The figure shows three views and two pictorial views of one solid part (mm, origin at its lowest corner). Answer the questions. A direction names the side the tool comes from. Coordinates: 2 decimals unless noted, no trailing zeros. Order: outer loops, then holes, each group sorted by start corner. A loop starts at its lowest first (then second) coordinate and runs counter-clockwise, first axis right, second up. Notation, with made-up numbers: (38, 80.5) - (54, 80.5) arc R18 cw to (54, 100.5) - close; hole circle Ø5 at (17.25, 86.25). An arc over 180 degrees is marked (long way). Answer as a JSON object with one key per item and string values. Group by question number.
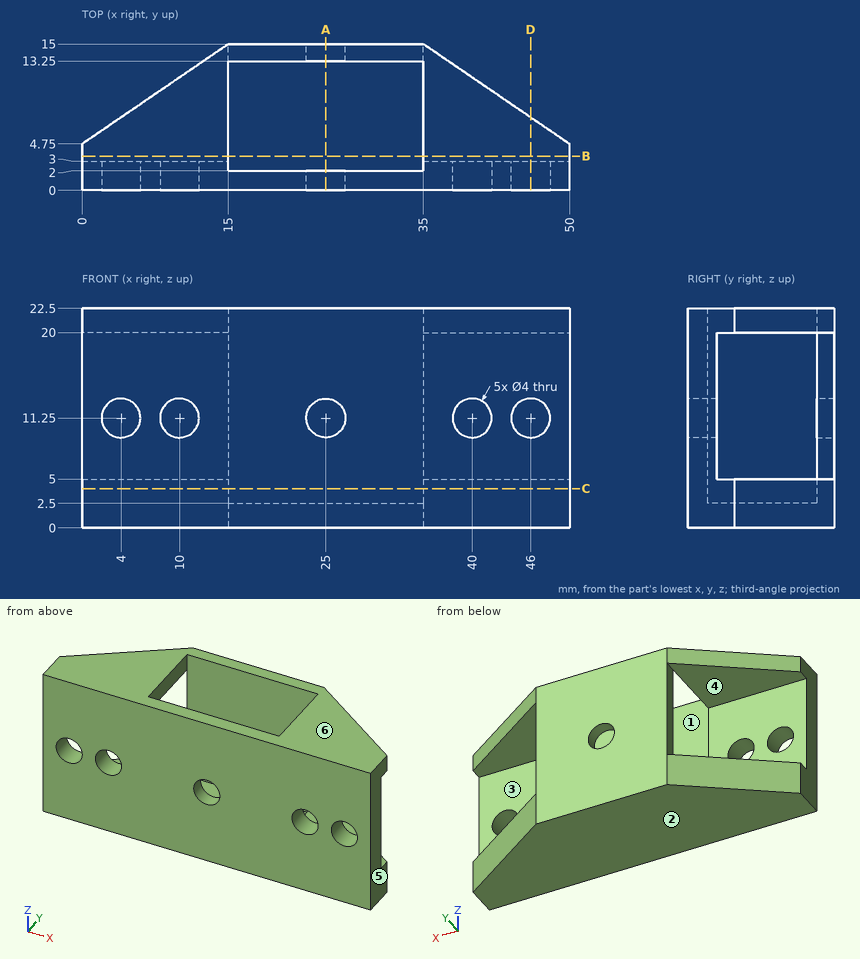
1. For the marked faces 1, 2 and 3, determine the directions among +Z, -Z, +X, -X, +Y, -Y from which every point of the face is accessible in a straight line to the end or side of a thin tool.
2. A cutting plane is placed at A-A on x = 25. Write down the section's boundary in (y, z), and give its area (3 significant figures).
3. A cutting plane is placed at B-B on y = 3.5. Write down the section's boundary in (x, z), and give its area (3 significant figures).
4. Straight lines are drawn through the part: L1, parallel to Z at x = 4, y = 1.4; L2, parallel to Z at x = 46, y = 5.75; L3, parallel to Y at x = 18, z = 8.5. For each, find the intervals that lie inside material, in ascending order.
5. Given pin 1 (12 mm diameter, centred on x = 42, z = 13, fed in from +Y); pin 2 (5.5 mm diameter, centred on y = 8.5, z = 11, fed in from -X); pin 3 (1.4 mm diameter, centred on y = 14.5, z = 14.5, fed in from +X); pin 4 (5.5 mm diameter, centred on x = 25.5, y = 5.5, fed in from +Z), each flat-ended and moving along its own axis, determine where each tip first touches the part or whether it passes through.
6. A cutting plane is placed at D-D on x = 46. Write down the section's boundary in (y, z).
7. For a pull along Z with two mould halves and no side action, classify the marked faces 4, 5 and 6 as pulls with the +Z half, pulls with the -Z half, needs draft (parallel to the pull), parting line crosses it, or undercut.
8. A cutting plane is placed at C-C on z = 4. Write down the section's boundary in (x, y).
Derived:
{
 "1": {"face 1": "+Z", "face 2": "-Z, +X, -X, +Y, -Y", "face 3": "+X, -X, +Y"},
 "2": {"outline": "(0, 0) - (15, 0) - (15, 9.25) - (13.25, 9.25) - (13.25, 2.5) - (2, 2.5) - (2, 9.25) - (0, 9.25) - close; (0, 13.25) - (2, 13.25) - (2, 22.5) - (0, 22.5) - close; (13.25, 13.25) - (15, 13.25) - (15, 22.5) - (13.25, 22.5) - close", "area": "97.5 mm2"},
 "3": {"outline": "(0, 0) - (50, 0) - (50, 5) - (35, 5) - (35, 2.5) - (15, 2.5) - (15, 5) - (0, 5) - close; (0, 20) - (15, 20) - (15, 22.5) - (0, 22.5) - close; (35, 20) - (50, 20) - (50, 22.5) - (35, 22.5) - close", "area": "275 mm2"},
 "4": {"L1": "z = 0 to 9.25, 13.25 to 22.5", "L2": "z = 0 to 5, 20 to 22.5", "L3": "y = 0 to 2, 13.25 to 15"},
 "5": {"pin 1": "stops at y = 3", "pin 2": "passes through", "pin 3": "stops at x = 35", "pin 4": "stops at z = 2.5"},
 "6": {"outline": "(0, 0) - (7.48, 0) - (7.48, 5) - (3, 5) - (3, 9.25) - (0, 9.25) - close; (0, 13.25) - (3, 13.25) - (3, 20) - (7.48, 20) - (7.48, 22.5) - (0, 22.5) - close"},
 "7": {"face 4": "undercut", "face 5": "needs draft", "face 6": "pulls with the +Z half"},
 "8": {"outline": "(0, 0) - (50, 0) - (50, 4.75) - (35, 15) - (15, 15) - (0, 4.75) - close; hole (15, 2) - (35, 2) - (35, 13.25) - (15, 13.25) - close"}
}
